Drawing for the job (mm, zero at the part's lowest x, y, z). A direction names the side the tool comes from. Give positions to 0.01 mm unless a question says otherwise; leave off trailing zeros. Write each loop counter-clockwise with the first axis right and the second up, starting at its lowest first coordinate (ties: lowest second). Pieces come first, ordered by that corner, then holes. Notation, with made-up numbers: M 71,77 L 104,77 A19 ccw 104,83 Z; hole C 52,-2.75 d7. An arc over 180 degrees is marked long. Answer as a JSON object with one key per item and string values. Group by question number.
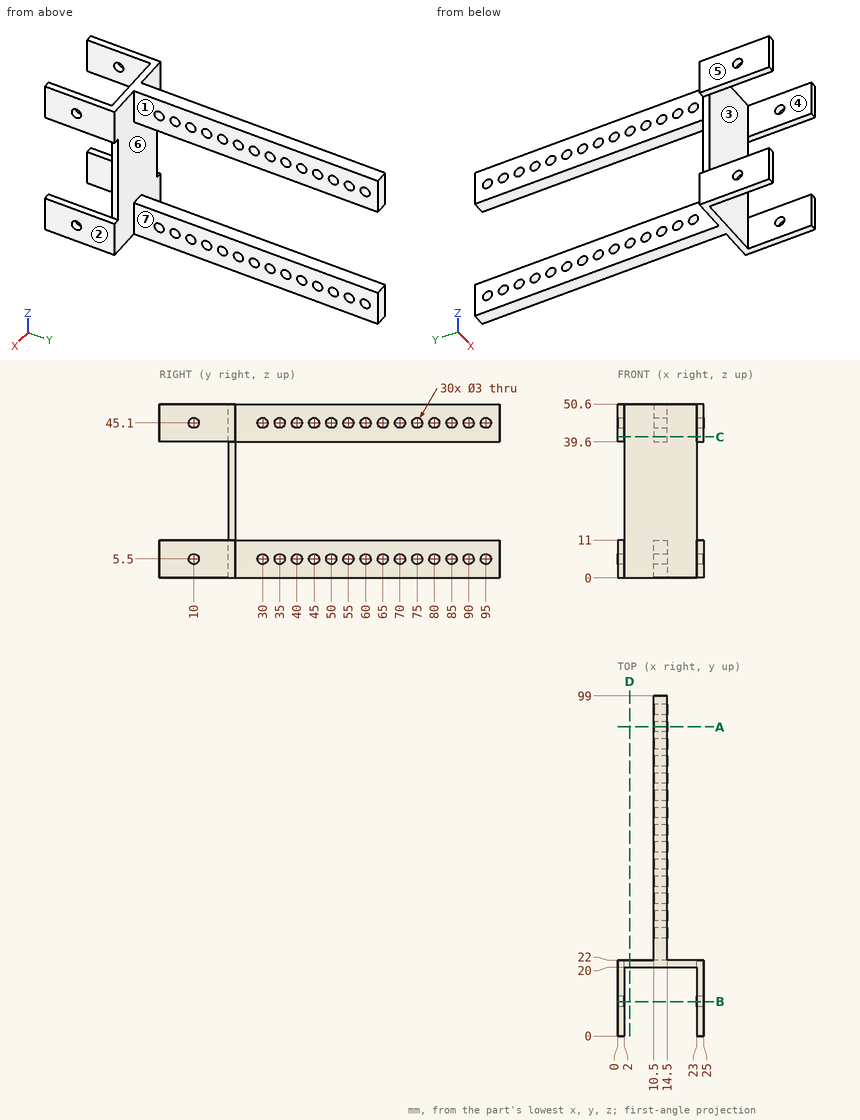
Q1. Slice it at B-B, the plane y = 10. Count the separate pieces of the cut face and the enclosed holes in it, then the cut area to 3 significant figures.
Q2. Wall check: L1, parallel to Z at x = 12.4, y = 95; L2, parallel to Z at x = 1.5, y = 17; L3, parallel to Y at x = 23.6, z = 5.5. Give the ranges that are in metal, low to high.
Q3. Slice it at A-A, the plane y = 90. Write the cut outline in (x, z).
Q4. 3-axis set-ups, long thin cutter, end or side, ignore diameter. For the marked faces 1, 2 and 3: which of +Z, -Z, +X, -X, +Y, -Y reach the whole face in a straight line?
Q5. Two-plate mould, pull along X, no slides. Class the marked faces 4, 5, 6 and 7: +X half, -X half, draft (parallel to the pull), parting line (faces both ways), or undercut.
Q6. Slice it at C-C, the plane z = 41. Write the cut outline in (x, y).
Q7. Slice it at D-D, the plane x = 3.5. Write the cut outline in (y, z).
Q8. Drop flat-ended pins along their axis: P1, Ø3.5, axis at y = 35, z = 5.5, coming from the +X side; P2, Ø8, axis at x = 15, z = 35.5, coming from the -Y side; P3, Ø5, axis at y = 34.5, z = 11.5, coming from the -X side. Give the stop position or say it passes through.
Solved:
{
 "1": {"separate pieces": "8", "enclosed holes": "0", "area": "64.0 mm²"},
 "2": {"L1": "z = 0 to 4, 7 to 11, 39.6 to 43.6, 46.6 to 50.6", "L2": "z = 0 to 11, 39.6 to 50.6", "L3": "y = 0 to 8.5, 11.5 to 22"},
 "3": {"outline": "M 10.5,0 L 14.5,0 L 14.5,4 L 10.5,4 Z; M 10.5,7 L 14.5,7 L 14.5,11 L 10.5,11 Z; M 10.5,39.6 L 14.5,39.6 L 14.5,43.6 L 10.5,43.6 Z; M 10.5,46.6 L 14.5,46.6 L 14.5,50.6 L 10.5,50.6 Z"},
 "4": {"face 1": "+Z, -Z, +X, +Y", "face 2": "+Z, -Z, +X, +Y, -Y", "face 3": "+Z, -Z, -Y"},
 "5": {"face 4": "undercut", "face 5": "-X half", "face 6": "draft", "face 7": "+X half"},
 "6": {"outline": "M 0,0 L 2,0 L 2,20 L 23,20 L 23,0 L 25,0 L 25,22 L 14.5,22 L 14.5,99 L 10.5,99 L 10.5,22 L 0,22 Z"},
 "7": {"outline": "M 20,0 L 22,0 L 22,50.6 L 20,50.6 Z"},
 "8": {"P1": "stops at x = 14.5", "P2": "stops at y = 20", "P3": "stops at x = 10.5"}
}
